Read the model definition and answer for the solid it produces. Units are mm, in the model's axes. Face numbers are marked on the shaded views. A direction names the side the tool comes from. Give positions to 0.01 mm unless a question says otherwise; leave off trailing zeros. Loops run counter-clockwise (first coordinate to the right, second up) from the corner with the lowest first, then second, coordinate; pieces in that order, holes last.
(1) Which of the six approach directions +Z, -Z, +X, -X, +Y, -Y give full straight-line access (tool end or side, diameter ignored) to the marked faces 4 and 5?
(2) Find section A-A, the plane x = 0. Write down the section's boundary in (y, z), then the cut area to 3 significant figures.
(3) Find section C-C, the plane z = 3.3. Write down the section's boundary in (x, y).
(4) Determine the mould class of the marked faces 1, 2 and 3 for opening direction X: pulls with the +X half, pulls with the -X half, needs draft (parallel to the pull), parting line crosses it, or undercut.
(5) Each of these flat-tipped pins is pushed along its axis until it touches: P1, Ø1, axis at x = -1, y = 0.5, coming from the -Z side; P2, Ø4.5, axis at x = 0, y = 0, coming from the -Z side. Where does it stop, or does it pass through?
(6) Straight lines are drawn through the part: probe 1 along Y at (x, z) = (0, 1.4); probe 2 along Z at (x, y) = (-3.25, 1); probe 3 along Y at (x, z) = (-0.5, 2.75). For each, find the intervals that lie inside material, in ascending order.
(7) Find section D-D, the plane y = -3.5. Write down the section's boundary in (x, z), then the cut area to 3 significant figures.
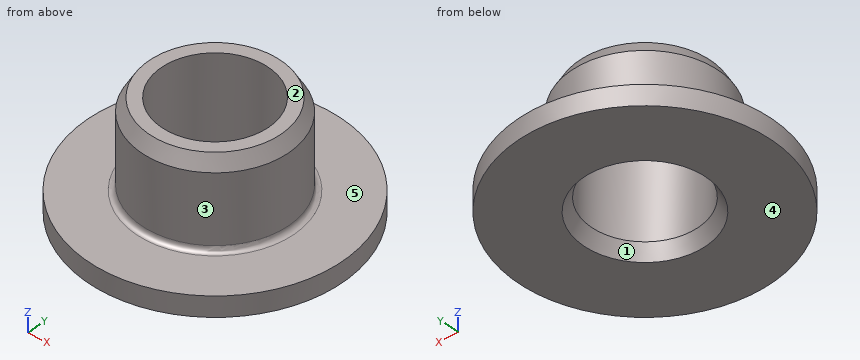
```python
from build123d import *

# Parameters (mm, degrees)
SKICA1_R        = 2.75
SKICA1_R_2      = 2
VYSUNOUT1_DEPTH = 4
SKICA2_R        = 4.75
SKICA2_R_2      = 2.75
VYSUNOUT2_DEPTH = 0.75
ZAOBLIT1_R      = 0.2
ZKOSIT1_SIZE    = 0.5
ZKOSIT1_SIZE2   = 0.288675135
ZKOSIT2_SIZE    = 0.288675135
ZKOSIT2_SIZE2   = 0.5


with BuildPart() as part:
    # Skica1 → Vysunout1 (new body)
    with BuildSketch(Plane.XY):
        Circle(SKICA1_R)
        Circle(SKICA1_R_2, mode=Mode.SUBTRACT)
    extrude(amount=VYSUNOUT1_DEPTH)

    # Skica2 → Vysunout2 (add)
    with BuildSketch(Plane(origin=(0, 0, 0), x_dir=(-1, 0, 0), z_dir=(0, 0, -1))):
        Circle(SKICA2_R)
        Circle(SKICA2_R_2, mode=Mode.SUBTRACT)
    extrude(amount=-VYSUNOUT2_DEPTH)

    # Zaoblit1
    zaoblit1_edges = [part.edges().sort_by_distance(p)[0] for p in [
        (-2.75, 0, 0.75),
    ]]
    fillet(zaoblit1_edges, radius=ZAOBLIT1_R)

    # Zkosit1
    zkosit1_edges = [part.edges().sort_by_distance(p)[0] for p in [
        (-2, 0, 0),
    ]]
    zkosit1_side = [part.faces().sort_by_distance(p)[0] for p in [
        (-2, 0, 2),
    ]]
    chamfer(zkosit1_edges, length=ZKOSIT1_SIZE, length2=ZKOSIT1_SIZE2, reference=zkosit1_side[0])

    # Zkosit2
    zkosit2_edges = [part.edges().sort_by_distance(p)[0] for p in [
        (-2.75, 0, 4),
    ]]
    zkosit2_side = [part.faces().sort_by_distance(p)[0] for p in [
        (-2.672218254, 0, 4),
    ]]
    chamfer(zkosit2_edges, length=ZKOSIT2_SIZE, length2=ZKOSIT2_SIZE2, reference=zkosit2_side[0])


solid = part.part
```
Entries:
1. face 4: -Z, +X, -X, +Y, -Y
1. face 5: +Z
2. outline: (-4.75, 0) - (-2.29, 0) - (-2, 0.5) - (-2, 4) - (-2.46, 4) - (-2.75, 3.5) - (-2.75, 0.95) arc R0.2 cw to (-2.95, 0.75) - (-4.75, 0.75) - close; (2, 0.5) - (2.29, 0) - (4.75, 0) - (4.75, 0.75) - (2.95, 0.75) arc R0.2 cw to (2.75, 0.95) - (2.75, 3.5) - (2.46, 4) - (2, 4) - close
2. area: 8.73 mm2
3. outline: circle Ø5.5 at (0, 0); hole circle Ø4 at (0, 0)
4. face 1: undercut
4. face 2: needs draft
4. face 3: parting line crosses it
5. P1: passes through
5. P2: stops at z = 0.07
6. probe 1: y = -2.75 to -2, 2 to 2.75
6. probe 2: z = 0 to 0.75
6. probe 3: y = -2.7 to -1.94, 1.94 to 2.7
7. outline: (-3.21, 0) - (3.21, 0) - (3.21, 0.75) - (-3.21, 0.75) - close
7. area: 4.82 mm2
